Design review of the part shown in the three views and the two pictorial views. Dimensions are in mm from the part's minimum x, y and z. A direction names the side the tool comes from. Give positions to 0.01 mm unless a question says otherwise; leave off trailing zeros. Loops run counter-clockwise (first coordinate to the right, second up) from the corner with the lowest first, then second, coordinate; pieces in that order, holes last.
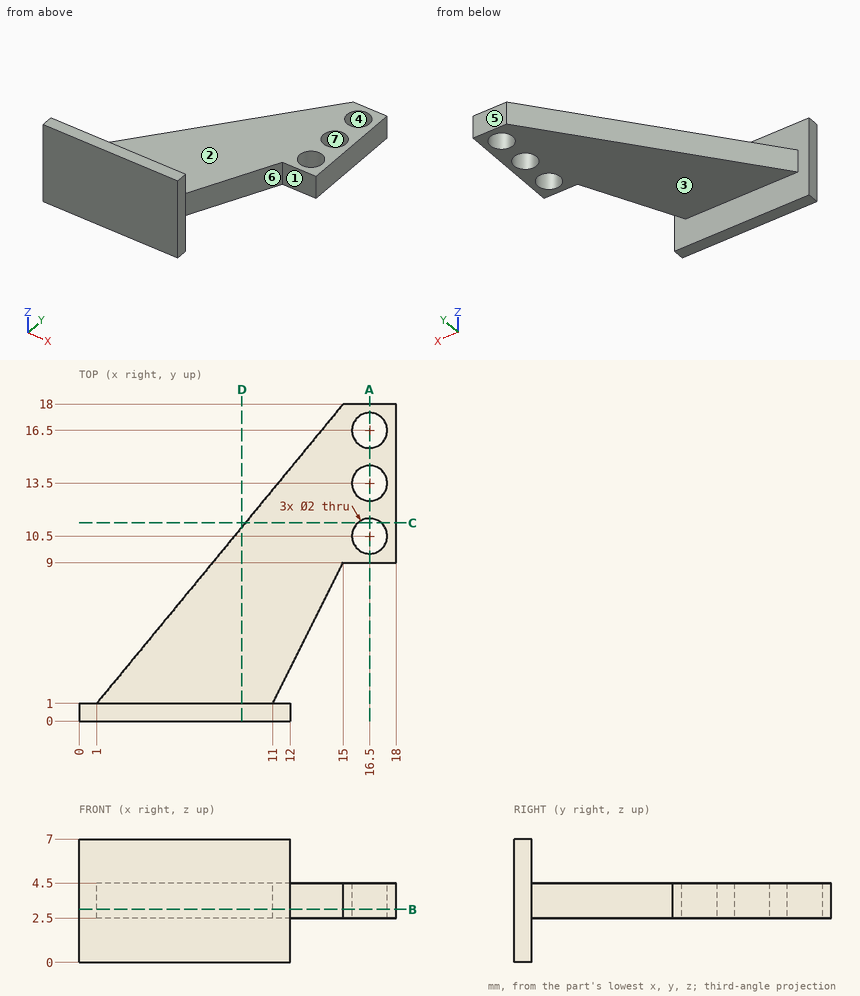
Q1. Consider section C-C on y = 11.25. Give the boundary of the cut face in (x, z), plus the area to 3 significant figures.
Answers:
outline: (9.44, 2.5) - (15.84, 2.5) - (15.84, 4.5) - (9.44, 4.5) - close; (17.16, 2.5) - (18, 2.5) - (18, 4.5) - (17.16, 4.5) - close
area: 14.5 mm2
Q2. For pin 1 Ø2 at (x, z) = (3, 3.5) entering from +Y; pin 2 Ø8 at (x, y) = (12, 2) entering from -Z; pin 3 Ø1 at (x, z) = (3, 1) entering from +Y; pin 4 Ø8 at (x, y) = (2, 12.5) entering from -Z, all flat-tipped, find the tip position at first contact; note any pin that passes through.
Answers:
pin 1: stops at y = 4.64
pin 2: stops at z = 0
pin 3: stops at y = 1
pin 4: passes through
Q3. For probe 1 along Y at (x, z) = (16.5, 3.6); probe 2 along Y at (x, z) = (3.75, 0.5); probe 3 along Z at (x, y) = (14.5, 13.5), list the stretches that pass through material, from the lowest coordinate up.
Answers:
probe 1: y = 9 to 9.5, 11.5 to 12.5, 14.5 to 15.5, 17.5 to 18
probe 2: y = 0 to 1
probe 3: z = 2.5 to 4.5
Q4. Mouldability with a two-part tool opening along X and no side actions: class the marked faces 5, 6 and 7 as +X half, -X half, draft (parallel to the pull), parting line (faces both ways), or undercut.
Answers:
face 5: draft
face 6: +X half
face 7: undercut
Q5. Machinability: for the marked faces 1, 2, 3 and 4, which of the approach directions +Z, -Z, +X, -X, +Y, -Y give a long, thin tool a straight path to every point of the face, cutting with its end or side? Answer none if there is none.
Answers:
face 1: +Z, -Z, +X, -Y
face 2: +Z, +X, -X, +Y
face 3: -Z, +X, -X, +Y
face 4: +Z, -Z
Q6. Consider section B-B on z = 3. Give the boundary of the cut face in (x, y).
Answers:
outline: (0, 0) - (12, 0) - (12, 1) - (11, 1) - (15, 9) - (18, 9) - (18, 18) - (15, 18) - (1, 1) - (0, 1) - close; hole circle Ø2 at (16.5, 10.5); hole circle Ø2 at (16.5, 13.5); hole circle Ø2 at (16.5, 16.5)
Q7. Consider section D-D on x = 9.25. Give the boundary of the cut face in (y, z), plus the area to 3 significant figures.
Answers:
outline: (0, 0) - (1, 0) - (1, 2.5) - (11.02, 2.5) - (11.02, 4.5) - (1, 4.5) - (1, 7) - (0, 7) - close
area: 27.0 mm2
Q8. Consider section A-A on x = 16.5. Give the boundary of the cut face in (y, z), plus the area to 3 significant figures.
Answers:
outline: (9, 2.5) - (9.5, 2.5) - (9.5, 4.5) - (9, 4.5) - close; (11.5, 2.5) - (12.5, 2.5) - (12.5, 4.5) - (11.5, 4.5) - close; (14.5, 2.5) - (15.5, 2.5) - (15.5, 4.5) - (14.5, 4.5) - close; (17.5, 2.5) - (18, 2.5) - (18, 4.5) - (17.5, 4.5) - close
area: 6.00 mm2
